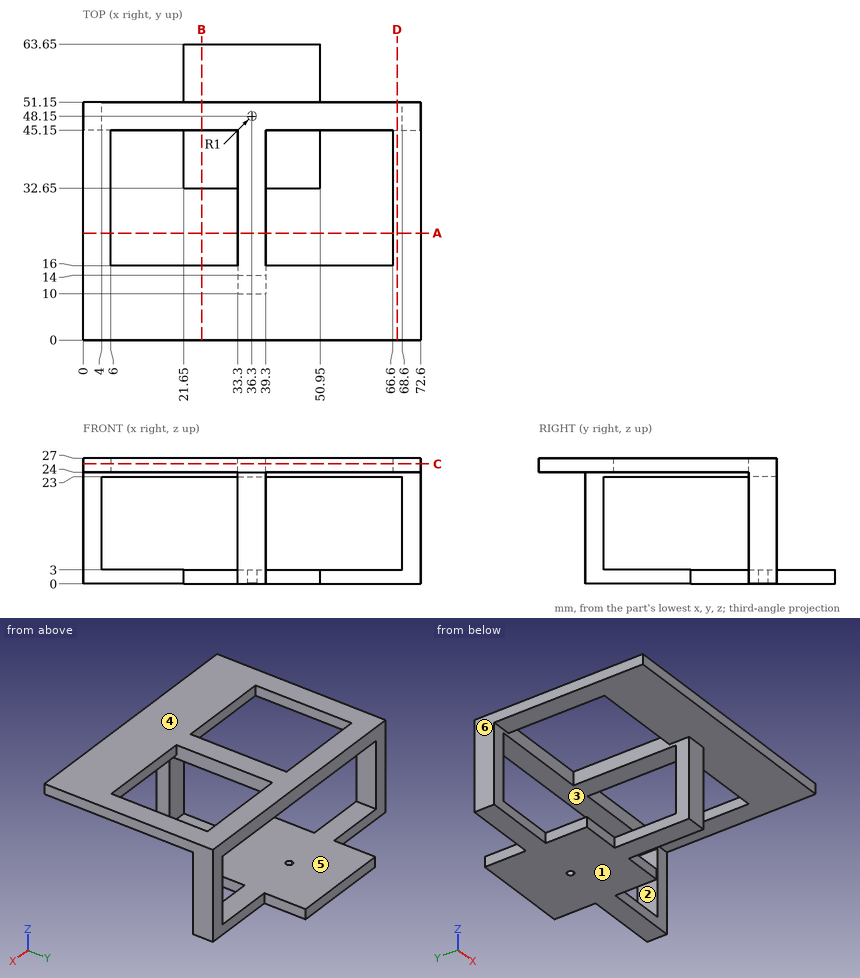
Geometry check sheet. Reference: drawing and pictorial views, mm from the part's lowest x, y, z. A direction names the side the tool comes from. Round coordinates to 2 decimals unless told otherwise and drop trailing zeros. Order: outer loops, then holes, each group sorted by start corner. A loop starts at its lowest first (then second) coordinate and runs counter-clockwise, first axis right, second up. Notation, with made-up numbers: (-29, 27.25) - (25, 27.25) arc R25 ccw to (25, 39.25) - close; hole circle Ø3 at (40, -32.75). An arc over 180 degrees is marked (long way). One line per question, with ' | ' between items. Start each with the question number.
(1) Release check for a two-part mould opening along Z. For the marked faces 4, 5 and 6 record: released by +Z, released by -Z, zero draft, split by the parting line, or undercut.
(2) Sectioned sample at A-A on y = 23. Record the cut outline in (x, z).
(3) Sectioned sample at D-D on x = 67.5. Record the cut outline in (y, z).
(4) Sectioned sample at B-B on x = 25.5. Record the cut outline in (y, z).
(5) Access from +Z, -Z, +X, -X, +Y, -Y to the whole of each face (thin tool, end or side, straight path). Record for the marked faces 1, 2 and 3.
(6) Sectioned sample at C-C on z = 25.75. Record the cut outline in (x, y), and give its area (3 significant figures).
(7) Depth check by flat-ended pin: pin 1 Ø3.5 at (y, z) = (37, 1) entering from +X; pin 2 Ø13.5 at (y, z) = (30.5, 14.5) entering from -X; pin 3 Ø1.5 at (x, z) = (29.5, 2) entering from -Y; pin 4 Ø2.5 at (y, z) = (41, 2) entering from -X. Enter the tip coordinate at first touch or a pass-through.
(8) Thickness scan on L1, parallel to X at y = 46, z = 14; L2, parallel to Y at x = 17, z = 25.75; L3, parallel to Z at x = 68.5, y = 48. Record the ranges inside material, lowest first. Write a range as [from, to].
Conclusion:
1) face 4: released by +Z | face 5: undercut | face 6: zero draft
2) outline: (0, 24) - (6, 24) - (6, 27) - (0, 27) - close; (33.3, 0) - (39.3, 0) - (39.3, 3) - (33.3, 3) - close; (33.3, 23) - (39.3, 23) - (39.3, 27) - (33.3, 27) - close; (66.6, 24) - (72.6, 24) - (72.6, 27) - (66.6, 27) - close
3) outline: (0, 24) - (45.15, 24) - (45.15, 23) - (51.15, 23) - (51.15, 27) - (0, 27) - close; (45.15, 0) - (51.15, 0) - (51.15, 3) - (45.15, 3) - close
4) outline: (0, 24) - (16, 24) - (16, 27) - (0, 27) - close; (32.65, 0) - (63.65, 0) - (63.65, 3) - (32.65, 3) - close; (45.15, 23) - (51.15, 23) - (51.15, 27) - (45.15, 27) - close
5) face 1: -Z, +X, -X, +Y, -Y | face 2: +Y, -Y | face 3: +Y
6) outline: (0, 0) - (72.6, 0) - (72.6, 51.15) - (0, 51.15) - close; hole (6, 16) - (33.3, 16) - (33.3, 45.15) - (6, 45.15) - close; hole (39.3, 16) - (66.6, 16) - (66.6, 45.15) - (39.3, 45.15) - close | area: 2,120 mm2
7) pin 1: stops at x = 50.95 | pin 2: passes through | pin 3: stops at y = 32.65 | pin 4: stops at x = 21.65
8) L1: x = [0, 4], [68.6, 72.6] | L2: y = [0, 16], [45.15, 51.15] | L3: z = [0, 3], [23, 27]
